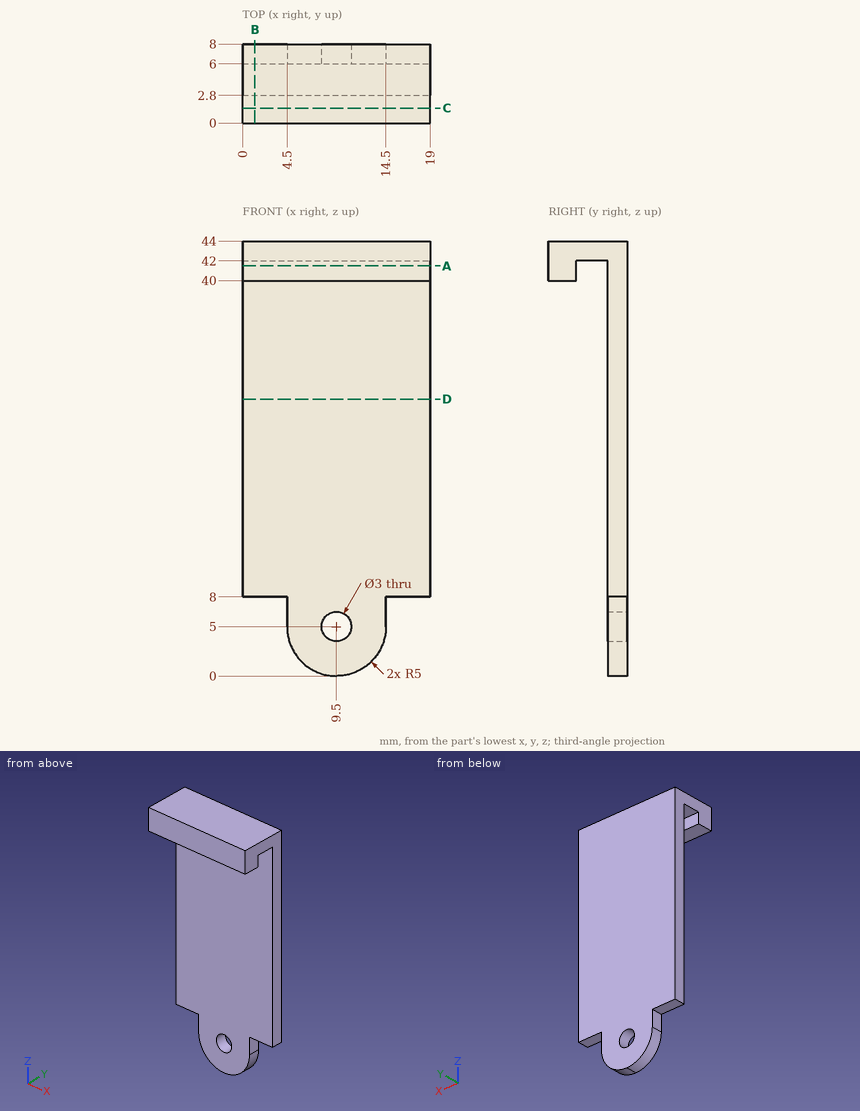
The drawing under review shows one solid part. Ordinate dimensions are in mm from its lowest x, y, z. Coordinates: 2 decimals unless noted, no trailing zeros. Write each loop counter-clockwise with the first axis right and the second up, starting at its lowest first coordinate (ties: lowest second). Pieces come first, ordered by that corner, then holes. Notation, with made-up numbers: (88.25, 81.25) -> (124.25, 81.25) arc R35 cw to (124.25, 119.25) -> close; hole circle Ø2 at (67, 67). An arc over 180 degrees is marked (long way). One line per item, written item: value. Start each with the question number.
Q1. Add section B-B, the plane x = 1.25. Give the boundary of the cut face in (y, z).
Q2. Add section C-C, the plane y = 1.5. Give the boundary of the cut face in (x, z), then the cut area to 3 significant figures.
Q3. Clearance check with flat-ended pins moving along their axes: P1, Ø3, axis at y = 5, z = 12.5, coming from the +X side; P2, Ø0.6, axis at y = 6.5, z = 7, coming from the -X side; P3, Ø1, axis at x = 16.5, y = 7, coming from the -Z side; P4, Ø1.6, axis at x = 8.5, y = 5, coming from the -Z side. State where each tip first meets the part, or that it passes through.
Q4. To check wall thickness, follow probe 1 along Z at (x, y) = (9.5, 6.45); probe 2 along X at (y, z) = (6.85, 5); probe 3 along Y at (x, z) = (8, 41). State the ranges of each line that lie inside material, in increasing order.
Q5. Add section A-A, the plane z = 41.5. Give the boundary of the cut face in (x, y).
Q6. Add section D-D, the plane z = 28. Give the boundary of the cut face in (x, y), then the cut area to 3 significant figures.
Response:
1. outline: (0, 40) -> (2.8, 40) -> (2.8, 42) -> (6, 42) -> (6, 8) -> (8, 8) -> (8, 44) -> (0, 44) -> close
2. outline: (0, 40) -> (19, 40) -> (19, 44) -> (0, 44) -> close
2. area: 76.0 mm²
3. P1: x = 19
3. P2: x = 4.5
3. P3: z = 8
3. P4: z = 42
4. probe 1: 0 to 3.5, 6.5 to 44
4. probe 2: 4.5 to 8, 11 to 14.5
4. probe 3: 0 to 2.8, 6 to 8
5. outline: (0, 0) -> (19, 0) -> (19, 2.8) -> (0, 2.8) -> close; (0, 6) -> (19, 6) -> (19, 8) -> (0, 8) -> close
6. outline: (0, 6) -> (19, 6) -> (19, 8) -> (0, 8) -> close
6. area: 38.0 mm²
